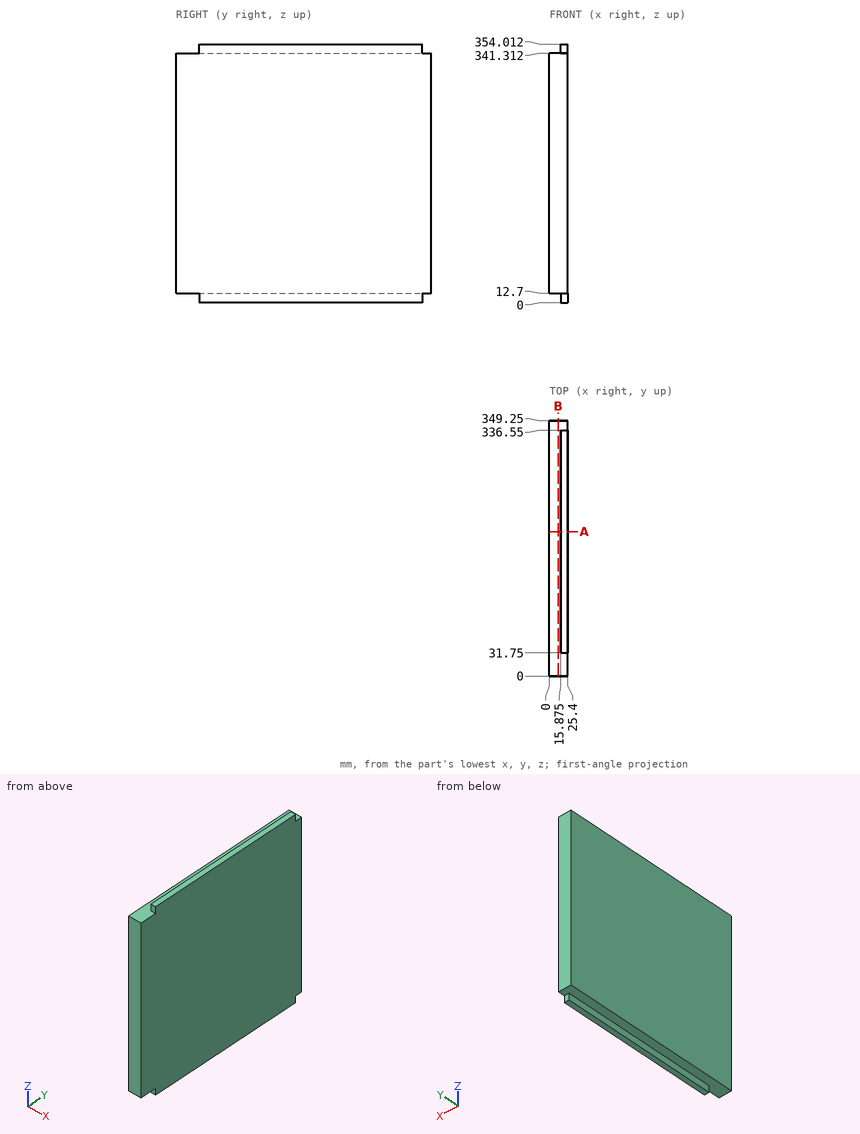
Geometry: see drawing. Coordinates: mm, zero at the bounding-box minimum. Round coordinates to 2 decimals unless told otherwise and drop trailing zeros. Write each loop counter-clockwise with the first axis right and the second up, starting at its lowest first coordinate (ties: lowest second). Pieces come first, ordered by that corner, then holes. Notation, with made-up numbers: M 37.25,-31.75 L 86.25,-31.75 A18 cw 86.25,-12.75 Z; hole C -10.5,5.5 d4. An arc over 180 degrees is marked long. Answer as a JSON object with one key per item and string values. Group by question number.
(1) Ray query, line 1 (Z direction, x = 18, y = 16). Return the intervals inside material, ascending. Write a range as [from, to].
(2) Section query B-B on x = 12. Output: boundary loops of the cut face in (y, z).
(3) Section query A-A on y = 197.5. Output: boundary loops of the cut face in (x, z) (1 decimal).
(4) First-contact query: pin 1 (10.5 mm diameter, centred on x = 22.5, z = 350, fed in from +Y); pin 2 (3 mm diameter, centred on x = 20, z = 7, fed in from -Y); pin 3 (14 mm diameter, centred on y = 247.5, z = 348.5, fed in from -X) (1 decimal). Flat tips, straight axial feed; report the tip coordinate or a pass-through.
Computed values:
{
 "1": {"line 1": "[12.7, 341.31]"},
 "2": {"outline": "M 0,12.7 L 349.25,12.7 L 349.25,341.31 L 0,341.31 Z"},
 "3": {"outline": "M 0,12.7 L 15.9,12.7 L 15.9,0 L 25.4,0 L 25.4,354 L 15.9,354 L 15.9,341.3 L 0,341.3 Z"},
 "4": {"pin 1": "y = 336.55", "pin 2": "y = 31.75", "pin 3": "x = 15.9"}
}
